For this review, take the finished solid that the model builds, in its own axes (mm). A direction names the side the tool comes from. Round coordinates to 2 decimals unless told otherwise and drop trailing zeros. Order: outer loops, then holes, each group sorted by start corner. A loop starts at its lowest first (then second) coordinate and runs counter-clockwise, first axis right, second up. Notation, with made-up numbers: (27.25, 31.25) - (85.25, 31.25) arc R21 ccw to (85.25, 57.25) - close; hole circle Ø2 at (54, -37.5). An arc over 180 degrees is marked (long way). One line per item, written item: value.
```python
from build123d import *

# Parameters (mm, degrees)
SKETCH6_R           = 31
BOSS_EXTRUDE3_DEPTH = 10
SKETCH7_R           = 3
CUT_EXTRUDE4_DEPTH  = 10
SKETCH8_R           = 2
BOSS_EXTRUDE8_DEPTH = 12


with BuildPart() as part:
    # Sketch6 → Boss-Extrude3 (new body)
    with BuildSketch(Plane(origin=(0, 0, 0), x_dir=(1, 0, 0), z_dir=(0, 1, 0))):
        with Locations(Location((0, 0, 0), (0, 0, 270))):
            Circle(SKETCH6_R)
    extrude(amount=BOSS_EXTRUDE3_DEPTH)

    # Sketch7 → Cut-Extrude4 (cut)
    with BuildSketch(Plane(origin=(0, 0, 0), x_dir=(1, 0, 0), z_dir=(0, 1, 0))):
        with Locations(Location((0, 26.248619222, 0), (0, 0, 270))):
            Circle(SKETCH7_R)
        with Locations(Location((26.123027742, 0, 0), (0, 0, 270))):
            Circle(SKETCH7_R)
        with Locations(Location((-24.615929988, 0, 0), (0, 0, 270))):
            Circle(SKETCH7_R)
        with Locations(Location((0, -26.248619222, 0), (0, 0, 270))):
            Circle(SKETCH7_R)
    extrude(amount=CUT_EXTRUDE4_DEPTH, mode=Mode.SUBTRACT)

    # Sketch8 → Boss-Extrude8 (add)
    with BuildSketch(Plane(origin=(0, 0, 0), x_dir=(1, 0, 0), z_dir=(0, 1, 0))):
        with BuildLine():
            Line((-38.449006602, -29.291772781), (29.291772781, 38.449006602))
            ThreePointArc((29.291772781, 38.449006602), (38.449006602, 38.449006602), (38.449006602, 29.291772781))
            Line((38.449006602, 29.291772781), (-29.291772781, -38.449006602))
            ThreePointArc((-29.291772781, -38.449006602), (-38.449006602, -38.449006602), (-38.449006602, -29.291772781))
        make_face()
        with Locations(Location((32.376246773, 32.540902219, 0), (0, 0, 270))):
            Circle(SKETCH8_R, mode=Mode.SUBTRACT)
        with Locations(Location((-32.456176129, -32.456176129, 0), (0, 0, 270))):
            Circle(SKETCH8_R, mode=Mode.SUBTRACT)
    extrude(amount=BOSS_EXTRUDE8_DEPTH)


solid = part.part
```
Item 1: Take a section at D-D (z = 0). Write out the cut boundary in (x, y), plus the area to 3 significant figures.
Returned:
outline: (-31, 0) - (-27.62, 0) - (-27.62, 10) - (-31, 10) - close; (-21.62, 0) - (23.12, 0) - (23.12, 10) - (9.16, 10) - (9.16, 12) - (-9.16, 12) - (-9.16, 10) - (-21.62, 10) - close; (29.12, 0) - (31, 0) - (31, 10) - (29.12, 10) - close
area: 537 mm^2
Item 2: For P1, Ø3, axis at x = -18.5, y = 4, coming from the +Z side; P2, Ø2, axis at y = 10, z = -12.5, coming from the -X side; P3, Ø5.5, axis at x = -24.62, z = 0, coming from the -Y side; P4, Ø6, axis at x = -18, y = 9, coming from the +Z side, all flat-tipped, find the tip position at first contact; note any pin that passes through.
Returned:
P1: z = 29.16
P2: x = -28.79
P3: through
P4: z = 30.16
Item 3: Machinability: for faces 4 (the flat face through (-5.053, 11.249, -4.104)), 5 (the flat face through (13, 10, 12)), 6 (the flat face through (-12, 10, -13)), which of the approach directions +Z, -Z, +X, -X, +Y, -Y give a long, thin tool a straight path to every point of the face, cutting with its end or side? Answer none if there is none.
Returned:
face 4: +Y
face 5: +Z, +X, +Y
face 6: -Z, -X, +Y
Item 4: Wall thickness on line 1 (X direction, y = 6.25, z = 0); line 2 (X direction, y = 5, z = -28); line 3 (Y direction, x = -13.5, z = 24.5): over which ranges is each line inside the solid? List them lowest first.
Returned:
line 1: -31 to -27.62, -21.62 to 23.12, 29.12 to 31
line 2: -13.3 to -2.44, 2.44 to 13.3, 18.84 to 37.16
line 3: 0 to 10
Item 5: Take a section at B-B (y = 3.5). Write out the cut boundary in (x, z).
Returned:
outline: (-38.45, 29.29) - (-26.02, 16.86) arc R31 ccw to (16.86, -26.02) - (29.29, -38.45) arc R6.48 ccw to (38.45, -29.29) - (26.02, -16.86) arc R31 ccw to (-16.86, 26.02) - (-29.29, 38.45) arc R6.48 ccw to start; hole circle Ø4 at (-32.46, 32.46); hole circle Ø6 at (-24.62, 0); hole circle Ø6 at (0, -26.25); hole circle Ø6 at (0, 26.25); hole circle Ø6 at (26.12, 0); hole circle Ø4 at (32.38, -32.54)
Item 6: Take a section at A-A (z = -27.5). Write out the cut boundary in (x, y).
Returned:
outline: (-14.31, 0) - (-2.73, 0) - (-2.73, 10) - (-14.31, 10) - close; (2.73, 0) - (14.31, 0) - (14.31, 10) - (2.73, 10) - close; (18.34, 0) - (36.66, 0) - (36.66, 12) - (18.34, 12) - close
Item 7: Take a section at C-C (x = 0). Write out the cut boundary in (y, z).
Returned:
outline: (0, -31) - (10, -31) - (10, -29.25) - (0, -29.25) - close; (0, -23.25) - (10, -23.25) - (10, -9.16) - (12, -9.16) - (12, 9.16) - (10, 9.16) - (10, 23.25) - (0, 23.25) - close; (0, 29.25) - (10, 29.25) - (10, 31) - (0, 31) - close
Item 8: The part is to be moulded in two halves that separate along X. For faces 1 (the flat face through (5.053, 11.249, 4.104)), 2 (the flat face through (1, 0, -1)), 3 (the cylindrical face through (38.347, 5.916, -38.549)), say which applies: +X half, -X half, draft (parallel to the pull), parting line (faces both ways), or undercut.
Returned:
face 1: undercut
face 2: draft
face 3: parting line
